```python
from build123d import *

# Parameters (mm, degrees)
F1_DEPTH = 5


with BuildPart() as f1:
    # F0 (on Front) → F1 (new body)
    with BuildSketch(Plane.XZ):
        with BuildLine():
            Line((14.079286, -2.855276), (7.309372, -0.148515))
            Line((7.309372, -0.148515), (6.311895, -3.230274))
            Line((6.311895, -3.230274), (8.425951, -2.590102))
            Line((8.425951, -2.590102), (11.090854, -3.140948))
            Line((11.090854, -3.140948), (12.609402, -4.510618))
            add(Edge.make_bspline(
                [(12.609402, -4.510618), (12.809735, -7.270896), (9.862116, -9.607936), (5.567014, -5.502325)],
                knots=[0, 0, 0, 0, 7.111871, 7.111871, 7.111871, 7.111871], degree=3))
            Line((5.567014, -5.502325), (4.788001, -8.113072))
            Line((4.788001, -8.113072), (4.184787, -12.078794))
            Line((4.184787, -12.078794), (3.954032, -16.039545))
            Line((3.954032, -16.039545), (6.276517, -14.520998))
            Line((6.276517, -14.520998), (8.837205, -14.163692))
            Line((8.837205, -14.163692), (11.189465, -15.846005))
            Line((11.189465, -15.846005), (11.695648, -18.689562))
            Line((11.695648, -18.689562), (9.641142, -22.753909))
            Line((9.641142, -22.753909), (5.231907, -27.910765))
            Line((5.231907, -27.910765), (0.20325, -32.395359))
            Line((0.20325, -32.395359), (1.997939, -32.792404))
            Line((1.997939, -32.792404), (13.096696, -25.990801))
            Line((13.096696, -25.990801), (19.260213, -20.154811))
            Line((19.260213, -20.154811), (22.982145, -13.366009))
            Line((22.982145, -13.366009), (25.572609, -6.1008))
            Line((25.572609, -6.1008), (25.840588, -2.855276))
            Line((25.840588, -2.855276), (27.436723, -1.431831))
            Line((27.436723, -1.431831), (27.947253, 0))
            Line((27.947253, 0), (23.964735, -2.408644))
            Line((23.964735, -2.408644), (19.915273, -3.123255))
            Line((19.915273, -3.123255), (14.079286, -2.855276))
        make_face()
    extrude(amount=F1_DEPTH)


solid = f1.part
```
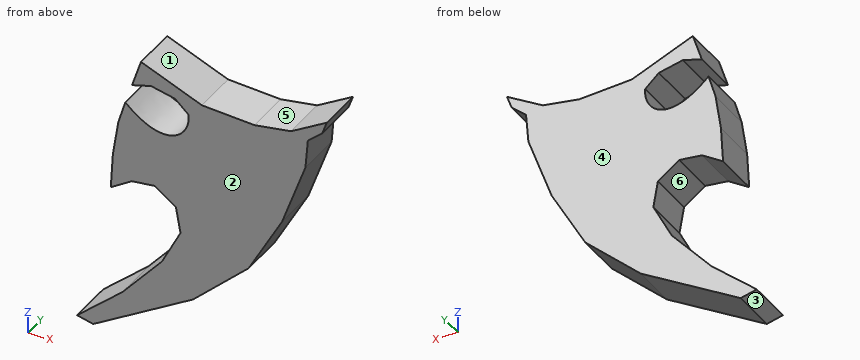
The listing builds one solid part. Answer for the finished solid, in the listing's coordinates (mm). Face numbers are marked on the shaded views. A direction names the side the tool comes from. Give positions to 0.01 mm unless a question says otherwise; leave off trailing zeros. Loops run counter-clockwise (first coordinate to the right, second up) from the corner with the lowest first, then second, coordinate; pieces in that order, holes last. Notation, with made-up numbers: M -7.75,78.5 L 39.25,78.5 A12 cw 39.25,85.5 Z; hole C -1,82 d11. An arc over 180 degrees is marked long. One line per item, written item: value.
1. Each of these flat-tipped pins is pushed along its axis until it touches: P1, Ø2, axis at y = -1.5, z = -19, coming from the +X side; P2, Ø1, axis at y = -4, z = -11.5, coming from the -X side; P3, Ø1.5, axis at x = 14, y = -3.5, coming from the +Z side. Where does it stop, or does it pass through?
Found:
P1: x = 20.44
P2: x = 4.2
P3: z = -2.52
2. For the marked faces 4, 5 and 6, determine the directions among +Z, -Z, +X, -X, +Y, -Y from which every point of the face is accessible in a straight line to the end or side of a thin tool.
Found:
face 4: +Z, -Z, +X, -X, +Y
face 5: +Z, +Y, -Y
face 6: +Y, -Y
3. For a pull along X with two mould halves and no side action, classify the marked faces 1, 2 and 3 as pulls with the +X half, pulls with the -X half, needs draft (parallel to the pull), parting line crosses it, or undercut.
Found:
face 1: undercut
face 2: needs draft
face 3: pulls with the -X half
4. Find the intervals of material crossed by probe 1 along Z at (x, y) = (10, -4.4); probe 2 along Z at (x, y) = (7.5, -0.85); probe 3 along X at (y, z) = (-2.15, -15.5), in increasing order.
Found:
probe 1: -27.89 to -22.04, -15 to -7.72, -2.92 to -1.22
probe 2: -29.42 to -25.26, -14.35 to -6.99, -2.87 to -0.22
probe 3: 3.99 to 4.78, 10.71 to 21.81
5. Section B-B on z = -16.5 is taken. Determine the outline of the cut face in (x, y).
Found:
outline: M 11.31,-5 L 21.26,-5 L 21.26,0 L 11.31,0 Z
6. Section A-A on x = 18.25 is taken. Determine the outline of the cut face in (y, z).
Found:
outline: M -5,-21.11 L 0,-21.11 L 0,-3.05 L -5,-3.05 Z
